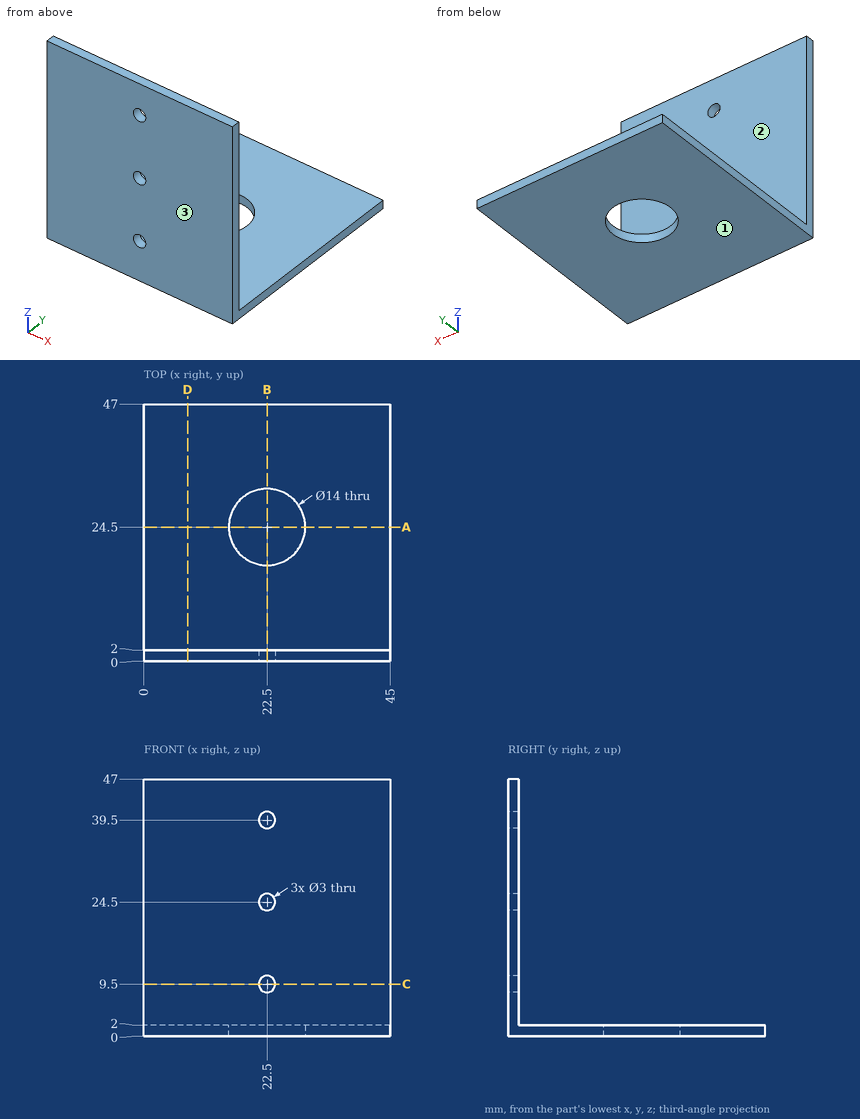
Verification items for this drawing (mm, ordinates from the low corner). Give positions to 0.01 mm unless a question says otherwise; leave off trailing zeros. Loops run counter-clockwise (first coordinate to the right, second up) from the corner with the lowest first, then second, coordinate; pieces in that order, holes last. Notation, with made-up numbers: M 69.5,74 L 74.5,74 A15 ccw 74.5,80 Z; hole C 62.25,-7 d2. An arc over 180 degrees is marked long. Return JSON: item names as keys, results as strings. Group by question number.
1. Go/stop test with flat-tipped pins: pin 1 (22.5 mm diameter, centred on x = 17.5, z = 19, fed in from +Y); pin 2 (1 mm diameter, centred on x = 7.5, y = 41.5, fed in from +Z). Record where each tip stops, or that it passes through.
2. Cross-section at B-B on x = 22.5. Record the boundary of the cut face in (y, z).
3. Cross-section at A-A on y = 24.5. Record the boundary of the cut face in (x, z), plus the area to 3 significant figures.
4. Cross-section at C-C on z = 9.5. Record the boundary of the cut face in (x, y), plus the area to 3 significant figures.
5. Mould release check, pull along Y, two halves, no side actions. Record for the marked faces 1, 2 and 3: released by +Y, released by -Y, zero draft, split by the parting line, or undercut.
6. Cross-section at D-D on x = 8. Record the boundary of the cut face in (y, z).
7. Thickness scan on L1, parallel to Z at x = 22.5, y = 0.8; L2, parallel to Y at x = 22.5, z = 1.05; L3, parallel to Y at x = 3, z = 3.5. Record the ranges inside material, lowest first.
Return value:
{
 "1": {"pin 1": "y = 2", "pin 2": "z = 2"},
 "2": {"outline": "M 0,0 L 17.5,0 L 17.5,2 L 2,2 L 2,8 L 0,8 Z; M 0,11 L 2,11 L 2,23 L 0,23 Z; M 0,26 L 2,26 L 2,38 L 0,38 Z; M 0,41 L 2,41 L 2,47 L 0,47 Z; M 31.5,0 L 47,0 L 47,2 L 31.5,2 Z"},
 "3": {"outline": "M 0,0 L 15.5,0 L 15.5,2 L 0,2 Z; M 29.5,0 L 45,0 L 45,2 L 29.5,2 Z", "area": "62.0 mm^2"},
 "4": {"outline": "M 0,0 L 21,0 L 21,2 L 0,2 Z; M 24,0 L 45,0 L 45,2 L 24,2 Z", "area": "84.0 mm^2"},
 "5": {"face 1": "zero draft", "face 2": "released by +Y", "face 3": "released by -Y"},
 "6": {"outline": "M 0,0 L 47,0 L 47,2 L 2,2 L 2,47 L 0,47 Z"},
 "7": {"L1": "0 to 8, 11 to 23, 26 to 38, 41 to 47", "L2": "0 to 17.5, 31.5 to 47", "L3": "0 to 2"}
}
